Read the model definition and answer for the solid it produces. Units are mm, in the model's axes. Face numbers are marked on the shaded views. A direction names the side the tool comes from. Coordinates: 2 decimals unless noted, no trailing zeros. Loops run counter-clockwise (first coordinate to the right, second up) from the corner with the lowest first, then second, coordinate; pieces in that order, holes last. Notation, with made-up numbers: M -30.75,60.5 L -15.75,60.5 A27 cw -15.75,96.5 Z; hole C 6.5,44 d5. An arc over 180 degrees is marked long. One line per item, written item: value. Start each with the question number.
1. Determine the mould class of the marked faces 3, 4, 5 and 6 for opening direction X: +X half, -X half, draft (parallel to the pull), parting line (faces both ways), or undercut.
2. The part is cut by section B-B (z = -233). Write down the section's boundary in (x, y).
3. Flat-ended cylindrical pins translate along their axes: pin 1 (4 mm diameter, centred on x = -105, z = 96, fed in from +Y); pin 2 (6 mm diameter, centred on x = 115.13, z = 341, fed in from +Y); pin 3 (7.5 mm diameter, centred on x = 69.13, z = 341, fed in from -Y). Find the tip coordinate at first contact, or state that the pin passes through.
4. For the marked faces 1 and 2, determine the directions among +Z, -Z, +X, -X, +Y, -Y from which every point of the face is accessible in a straight line to the end or side of a thin tool.
5. The part is cut by section A-A (y = 325). Write down the section's boundary in (x, z), then the cut area to 3 significant figures.
6. Consider probe 1 along X at (y, z) = (216.5, 227); probe 2 along Z at (x, y) = (184, 310.5); probe 3 along Y at (x, z) = (63, 264). Determine where each line is inside the solid, lowest interval first.
7. The part is cut by section C-C (x = -100). Write down the section's boundary in (y, z), then the cut area to 3 significant figures.
```python
from build123d import *

# Parameters (mm, degrees)
TABAN_FLAN_1_DEPTH    = 400
IZIM6_R               = 3.25
KES_EKSTR_ZYON1_DEPTH = 10
IZIM7_R               = 4.25
KES_EKSTR_ZYON2_DEPTH = 10


# Sheet-metal steps are written as plain solids
with BuildPart() as part:
    # Çizim1 → Taban-Flanş1 (new, symmetric)
    with BuildSketch(Plane.XY):
        with BuildLine():
            Line((-185, 420), (-185, 2.5))
            ThreePointArc((-185, 2.5), (-184.267766953, 0.732233047), (-182.5, 0))
            Line((-182.5, 0), (182.5, 0))
            ThreePointArc((182.5, 0), (184.267766953, 0.732233047), (185, 2.5))
            Line((185, 2.5), (185, 420))
            Line((185, 420), (183.5, 420))
            Line((183.5, 420), (183.5, 2.5))
            ThreePointArc((183.5, 2.5), (183.207106781, 1.792893219), (182.5, 1.5))
            Line((182.5, 1.5), (-182.5, 1.5))
            ThreePointArc((-182.5, 1.5), (-183.207106781, 1.792893219), (-183.5, 2.5))
            Line((-183.5, 2.5), (-183.5, 420))
            Line((-183.5, 420), (-185, 420))
        make_face()
    extrude(amount=TABAN_FLAN_1_DEPTH, both=True)

    # Çizim6 → Kes-Ekstrüzyon1 (cut)
    with BuildSketch(Plane.XZ):
        with Locations((-115.125314072, 341)):
            Circle(IZIM6_R)
        with Locations((-69.125314072, 341)):
            Circle(IZIM6_R)
        with Locations((69.125314072, 341)):
            Circle(IZIM6_R)
        with Locations((115.125314072, 341)):
            Circle(IZIM6_R)
        with Locations((115.125314072, -341)):
            Circle(IZIM6_R)
        with Locations((69.125314072, -341)):
            Circle(IZIM6_R)
        with Locations((-69.125314072, -341)):
            Circle(IZIM6_R)
        with Locations((-115.125314072, -341)):
            Circle(IZIM6_R)
    extrude(amount=-KES_EKSTR_ZYON1_DEPTH, mode=Mode.SUBTRACT)

    # Çizim7 → Kes-Ekstrüzyon2 (cut)
    with BuildSketch(Plane(origin=(185, 0, 0), x_dir=(0, 0, -1), z_dir=(1, 0, 0))):
        with Locations(Location((-300, 310.5, 0), (0, 0, 90))):
            Circle(IZIM7_R)
        with Locations(Location((-300, 196.5, 0), (0, 0, 90))):
            Circle(IZIM7_R)
        with Locations(Location((300, 196.5, 0), (0, 0, 90))):
            Circle(IZIM7_R)
        with Locations(Location((300, 310.5, 0), (0, 0, 90))):
            Circle(IZIM7_R)
    extrude(amount=-KES_EKSTR_ZYON2_DEPTH, mode=Mode.SUBTRACT)


solid = part.part
```
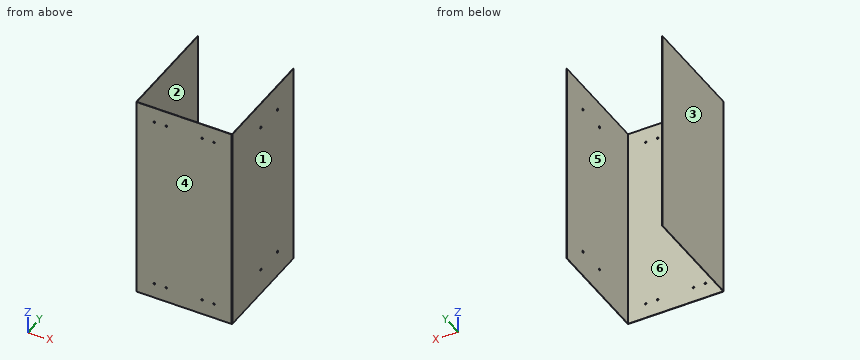
Answer block:
1. face 3: -X half
1. face 4: draft
1. face 5: undercut
1. face 6: undercut
2. outline: M -185,2.5 A2.5 ccw -182.5,0 L 182.5,0 A2.5 ccw 185,2.5 L 185,420 L 183.5,420 L 183.5,2.5 A1 cw 182.5,1.5 L -182.5,1.5 A1 cw -183.5,2.5 L -183.5,420 L -185,420 Z
3. pin 1: stops at y = 1.5
3. pin 2: passes through
3. pin 3: stops at y = 0
4. face 1: +Z, -Z, +X, +Y, -Y
4. face 2: +Z, -Z, +Y
5. outline: M -185,-400 L -183.5,-400 L -183.5,400 L -185,400 Z; M 183.5,-400 L 185,-400 L 185,400 L 183.5,400 Z
5. area: 2,400 mm2
6. probe 1: x = -185 to -183.5, 183.5 to 185
6. probe 2: z = -400 to -304.25, -295.75 to 295.75, 304.25 to 400
6. probe 3: y = 0 to 1.5
7. outline: M 0,-400 L 1.5,-400 L 1.5,400 L 0,400 Z
7. area: 1,200 mm2
